The model under review builds one solid part; all positions refer to its coordinate system, in mm. Round coordinates to 2 decimals unless told otherwise and drop trailing zeros. Loops run counter-clockwise (first coordinate to the right, second up) from the corner with the lowest first, then second, coordinate; pieces in that order, holes last. Notation, with made-up numbers: (-5.75, 68.25) -> (21.25, 68.25) arc R38 cw to (21.25, 106.25) -> close; hole circle Ø4 at (86, -11.5). An arc over 180 degrees is marked (long way). Use CSV: the item, a comma, the result in double quotes. Start each with the question number.
```python
from build123d import *

# Parameters (mm, degrees)
SKETCH1_R           = 1.5
SKETCH1_R_2         = 2.5
BOSS_EXTRUDE1_DEPTH = 8


with BuildPart() as part:
    # Sketch1 → Boss-Extrude1 (new body)
    with BuildSketch(Plane(origin=(0, 0, 0), x_dir=(1, 0, 0), z_dir=(0, 1, 0))):
        Polygon((-8.795, -36.47), (8.795, -36.47), (25.001887425, -20.263112575), (25.001887425, -7.783112575), (15.88249732, 17.378899724), (-15.88249732, 17.378899724), (-25.001887425, -7.783112575), (-25.001887425, -20.263112575), align=None)
        with Locations((-5, 0)):
            Circle(SKETCH1_R, mode=Mode.SUBTRACT)
        with Locations((5, 0)):
            Circle(SKETCH1_R, mode=Mode.SUBTRACT)
        with Locations((0, -20)):
            Circle(SKETCH1_R_2, mode=Mode.SUBTRACT)
        with Locations((12.37637727, 12.378899724)):
            Circle(SKETCH1_R, mode=Mode.SUBTRACT)
        with Locations((-12.37637727, 12.378899724)):
            Circle(SKETCH1_R, mode=Mode.SUBTRACT)
    extrude(amount=BOSS_EXTRUDE1_DEPTH)


solid = part.part
```
1. Take a section at C-C, the plane y = 6.25. Give the boundary of the cut face in (x, z) (1 decimal), then the cut area to 3 significant figures.
2. The part is to be moulded in two halves that separate along X. For faces 1 (the face through (25.002, 4, 14)), 2 (the face through (0, 4, 36.47)), 3 (the face through (13.183, 3.944, -13.644)), say which applies: pulls with the +X half, pulls with the -X half, needs draft (parallel to the pull), parting line crosses it, or undercut.
3. Take a section at A-A, the plane x = 0. Give the boundary of the cut face in (y, z).
4. For line 1 along X through (y, z) = (3, 20); line 2 along X through (y, z) = (5, 0); line 3 along Z through (x, y) = (5, 2.5), list the stretches that pass through material, from the lowest coordinate up. Write a range as from..to.
5. Take a section at D-D, the plane x = -11.5. Give the boundary of the cut face in (y, z) (3 decimals), then the cut area to 3 significant figures.
6. Take a section at B-B, the plane z = 0. Give the boundary of the cut face in (x, y), then the cut area to 3 significant figures.
Results:
1,outline,"(-25, 7.8) -> (-15.9, -17.4) -> (15.9, -17.4) -> (25, 7.8) -> (25, 20.3) -> (8.8, 36.5) -> (-8.8, 36.5) -> (-25, 20.3) -> close; hole circle Ø3 at (-12.4, -12.4); hole circle Ø3 at (-5, 0); hole circle Ø5 at (0, 20); hole circle Ø3 at (5, 0); hole circle Ø3 at (12.4, -12.4)"
1,area,"2,150 mm²"
2,face 1,"pulls with the +X half"
2,face 2,"needs draft"
2,face 3,"undercut"
3,outline,"(0, -17.38) -> (8, -17.38) -> (8, 17.5) -> (0, 17.5) -> close; (0, 22.5) -> (8, 22.5) -> (8, 36.47) -> (0, 36.47) -> close"
4,line 1,"-25..-2.5, 2.5..25"
4,line 2,"-22.18..-6.5, -3.5..3.5, 6.5..22.18"
4,line 3,"-17.38..-1.5, 1.5..36.47"
5,outline,"(0, -17.379) -> (8, -17.379) -> (8, -13.596) -> (0, -13.596) -> close; (0, -11.162) -> (8, -11.162) -> (8, 33.765) -> (0, 33.765) -> close"
5,area,"390 mm²"
6,outline,"(-22.18, 0) -> (-6.5, 0) -> (-6.5, 8) -> (-22.18, 8) -> close; (-3.5, 0) -> (3.5, 0) -> (3.5, 8) -> (-3.5, 8) -> close; (6.5, 0) -> (22.18, 0) -> (22.18, 8) -> (6.5, 8) -> close"
6,area,"307 mm²"
